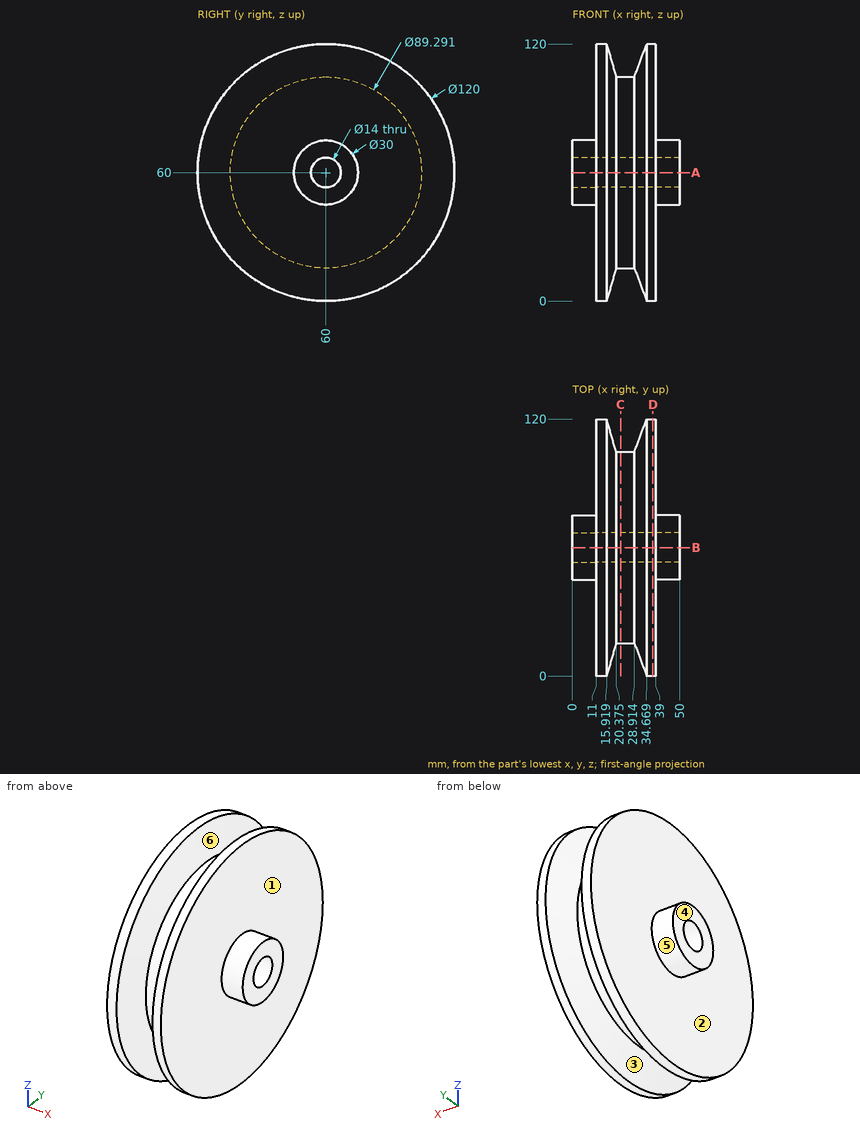
The figure shows three views and two pictorial views of one solid part (mm, origin at its lowest corner). Answer the questions. A direction names the side the tool comes from. Coordinates: 2 decimals unless noted, no trailing zeros. Loops run counter-clockwise (first coordinate to the right, second up) from the corner with the lowest first, then second, coordinate; pieces in that order, holes last.
1) A tool of negligible diameter and unlimited length cuts with its end or side. For the marked faces 1, 2 and 3, from which of +Z, -Z, +X, -X, +Y, -Y can it reach the whole face along a straight path? Write none if from no direction.
2) Find section A-A on z = 60. Write down the section's boundary in (x, y) (1 decimal).
3) Find the intervals of material crossed by L1, parallel to Y at x = 23.5, z = 60 (1 decimal); L2, parallel to Y at x = 5, z = 60; L3, parallel to Z at x = 36.5, y = 60, in increasing order.
4) Determine the mould class of the marked faces 4, 5 and 6 for opening direction X: pulls with the +X half, pulls with the -X half, needs draft (parallel to the pull), parting line crosses it, or undercut.
5) Flat-ended cylindrical pins translate along their axes: pin 1 Ø6 at (x, y) = (41.5, 30) entering from -Z (1 decimal); pin 2 Ø4 at (x, y) = (40, 42.5) entering from -Z; pin 3 Ø3 at (x, y) = (38, 22.5) entering from -Z. Find the tip coordinate at first contact, or state that the pin passes through.
6) Find section D-D on x = 37.5. Write down the section's boundary in (y, z).
7) Find section C-C on x = 22.5. Write down the section's boundary in (y, z) (1 decimal).
Values:
1. face 1: +X
1. face 2: -X
1. face 3: none
2. outline: (0, 45) - (11, 45) - (11, 0) - (15.9, 0) - (20.4, 15.4) - (28.9, 15.4) - (34.7, 0) - (39, 0) - (39, 45) - (50, 45) - (50, 53) - (0, 53) - close; (0, 67) - (50, 67) - (50, 75) - (39, 75) - (39, 120) - (34.7, 120) - (28.9, 104.6) - (20.4, 104.6) - (15.9, 120) - (11, 120) - (11, 75) - (0, 75) - close
3. L1: y = 15.4 to 53, 67 to 104.6
3. L2: y = 45 to 53, 67 to 75
3. L3: z = 0 to 53, 67 to 120
4. face 4: pulls with the -X half
4. face 5: needs draft
4. face 6: undercut
5. pin 1: stops at z = 7.1
5. pin 2: stops at z = 2.11
5. pin 3: stops at z = 12
6. outline: circle Ø120 at (60, 60); hole circle Ø14 at (60, 60)
7. outline: circle Ø89.3 at (60, 60); hole circle Ø14 at (60, 60)
